Can you work these out from the drawing? Everything is in mm from the part's minimum corner. A direction names the side the tool comes from. Round coordinates to 2 decimals unless told otherwise and drop trailing zeros. Loops run counter-clockwise (first coordinate to the right, second up) from the corner with the lowest first, then second, coordinate; pieces in that order, holes last. Notation, with made-up numbers: M -18,74.5 L -14,74.5 A18 cw -14,82.5 Z; hole C 46,-2 d5. An arc over 180 degrees is marked long. Return JSON: item names as keys, results as strings. Group by question number.
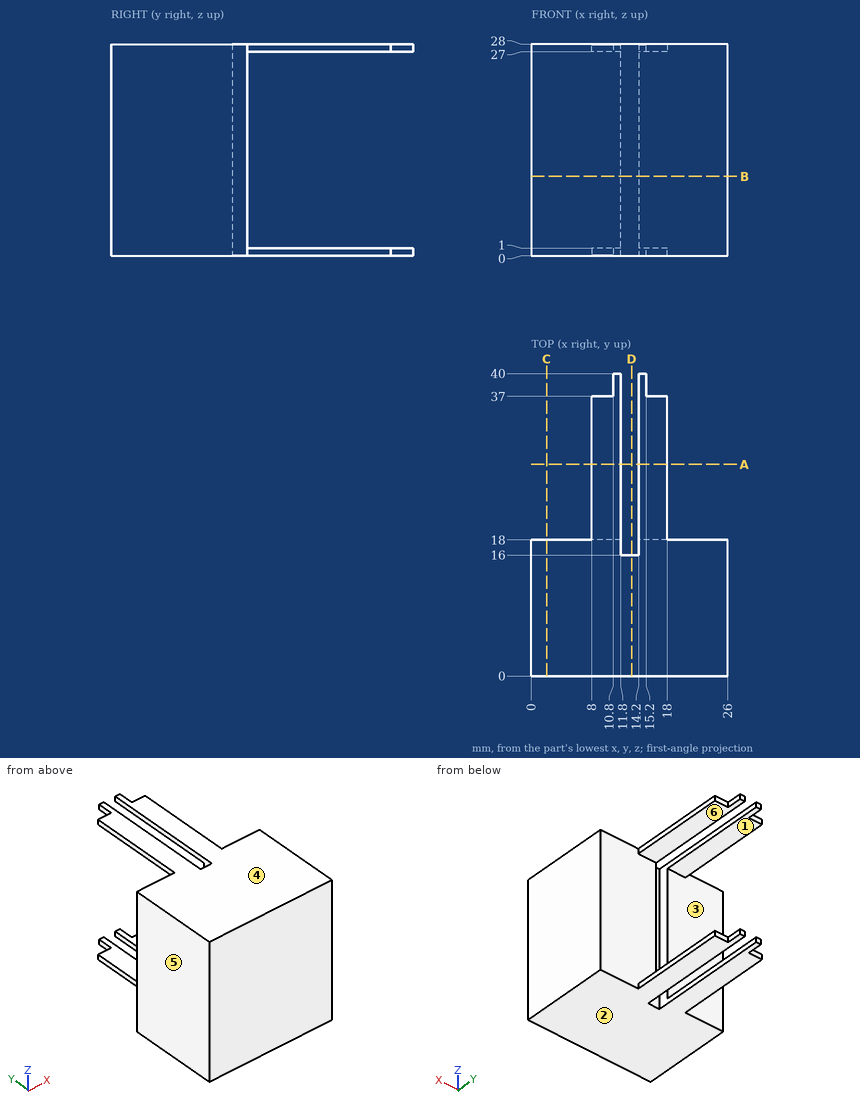
1. If we section it at D-D, the plane x = 13.25: Please give me the cut outline in (y, z), then the cut area to 3 significant figures.
2. If we section it at C-C, the plane x = 2: Please give me the cut outline in (y, z), then the cut area to 3 significant figures.
3. We'd pull the mould along Z, two halves only. Please class the marked faces 3, 4, 5 and 6: +Z half, -Z half, draft (parallel to the pull), parting line (faces both ways), or undercut.
4. On a 3-axis mill with a long thin cutter (end or side, diameter ignored), from which of +Z, -Z, +X, -X, +Y, -Y can I reach the whole of each face in a straight line? I mean the marked faces 1 and 2. Say none if no direction works.
5. If we section it at B-B, the plane z = 10.5: Please give me the cut outline in (x, y).
6. If we section it at A-A, the plane y = 28: Please give me the cut outline in (x, z), then the cut area to 3 significant figures.
7. I'm going to push flat-ended pins straight in: pin 1 Ø0.5 at (x, z) = (16.5, 27.5) entering from +Y; pin 2 Ø2 at (x, y) = (19.5, 29) entering from -Z; pin 3 Ø0.8 at (y, z) = (28, 0.5) entering from -X; pin 4 Ø10 at (x, z) = (3, 25) entering from +Y. Where does each tip first touch, or does it pass through?
8. I need wall thicknesses on probe 1 along Z at (x, y) = (16.5, 29.5); probe 2 along Y at (x, z) = (1, 6.25); probe 3 along Y at (x, z) = (14, 8). Which ranges of each line are inside material? Lowest first, please.
Geometry results:
{
 "1": {"outline": "M 0,0 L 16,0 L 16,28 L 0,28 Z", "area": "448 mm^2"},
 "2": {"outline": "M 0,0 L 18,0 L 18,28 L 0,28 Z", "area": "504 mm^2"},
 "3": {"face 3": "undercut", "face 4": "+Z half", "face 5": "draft", "face 6": "undercut"},
 "4": {"face 1": "+X, -X, +Y", "face 2": "-Z, +X, -X, +Y, -Y"},
 "5": {"outline": "M 0,0 L 26,0 L 26,18 L 14.2,18 L 14.2,16 L 11.8,16 L 11.8,18 L 0,18 Z"},
 "6": {"outline": "M 8,0 L 11.8,0 L 11.8,1 L 8,1 Z; M 8,27 L 11.8,27 L 11.8,28 L 8,28 Z; M 14.2,0 L 18,0 L 18,1 L 14.2,1 Z; M 14.2,27 L 18,27 L 18,28 L 14.2,28 Z", "area": "15.2 mm^2"},
 "7": {"pin 1": "y = 37", "pin 2": "through", "pin 3": "x = 8", "pin 4": "y = 18"},
 "8": {"probe 1": "0 to 1, 27 to 28", "probe 2": "0 to 18", "probe 3": "0 to 16"}
}
